from build123d import *

# Parameters (mm, degrees)
CUT_EXTRUDE1_START    = 5.5
CUT_EXTRUDE1_DEPTH    = 10
SKETCH8_R             = 6
CUT_EXTRUDE4_DEPTH    = 6
CUT_EXTRUDE5_START    = 6
CUT_EXTRUDE5_DEPTH    = 2.5
FILLET1_R             = 0.3
CHAMFER1_SIZE         = 0.5
M3_TAPPED_HOLE1_D     = 2.5
M3_TAPPED_HOLE1_DEPTH = 6.748924226
M3_TAPPED_HOLE1_TIP   = 0.751075774


with BuildPart() as part:
    # Sketch3 → Revolve1 (revolve)
    with BuildSketch(Plane.XY):
        Polygon((-10, 9), (10, 9), (10, 6), (32, 6), (60, 6), (60, 0), (-30, 0), (-30, 6), (-10, 6), align=None)
    revolve(axis=Axis((-30, 0, 0), (1, 0, 0)))

    # Sketch5 → Cut-Extrude1 (cut)
    with BuildSketch(Plane(origin=(0, 0, 0), x_dir=(1, 0, 0), z_dir=(0, 1, 0)).offset(CUT_EXTRUDE1_START)):
        with BuildLine():
            Line((5, -3), (-5, -3))
            ThreePointArc((-5, -3), (-8, 0), (-5, 3))
            Line((-5, 3), (5, 3))
            ThreePointArc((5, 3), (8, 0), (5, -3))
        make_face()
    extrude(amount=CUT_EXTRUDE1_DEPTH, mode=Mode.SUBTRACT)

    # Sketch8 → Cut-Extrude4 (cut)
    with BuildSketch(Plane(origin=(60, 0, 0), x_dir=(0, 0, -1), z_dir=(1, 0, 0))):
        Circle(SKETCH8_R)
    extrude(amount=-CUT_EXTRUDE4_DEPTH, mode=Mode.SUBTRACT)

    # Sketch9 → Cut-Extrude5 (cut)
    with BuildSketch(Plane(origin=(0, 0, 0), x_dir=(1, 0, 0), z_dir=(0, 1, 0)).offset(CUT_EXTRUDE5_START)):
        with BuildLine():
            Line((42, 2), (48, 2))
            ThreePointArc((48, 2), (50, 0), (48, -2))
            Line((48, -2), (42, -2))
            ThreePointArc((42, -2), (40, 0), (42, 2))
        make_face()
    extrude(amount=-CUT_EXTRUDE5_DEPTH, mode=Mode.SUBTRACT)

    # Fillet1
    fillet1_edges = [part.edges().sort_by_distance(p)[0] for p in [
        (-10, -6, 0),
        (10, -6, 0),
    ]]
    fillet(fillet1_edges, radius=FILLET1_R)

    # Chamfer1
    chamfer1_edges = [part.edges().sort_by_distance(p)[0] for p in [
        (-30, -6, 0),
        (54, -6, 0),
    ]]
    chamfer(chamfer1_edges, length=CHAMFER1_SIZE)

    # M3 Tapped Hole1
    with Locations(Plane(origin=(54, 0, 0), x_dir=(0, 0, -1), z_dir=(1, 0, 0))):
        with Locations((0, 0)):
            Hole(M3_TAPPED_HOLE1_D / 2, depth=M3_TAPPED_HOLE1_DEPTH)
            with Locations((0, 0, -(M3_TAPPED_HOLE1_DEPTH + M3_TAPPED_HOLE1_TIP / 2))):  # 118° drill point
                Cone(0, M3_TAPPED_HOLE1_D / 2, M3_TAPPED_HOLE1_TIP, mode=Mode.SUBTRACT)


solid = part.part
The model under review builds one solid part; all positions refer to its coordinate system, in mm. A direction names the side the tool comes from. Round coordinates to 2 decimals unless told otherwise and drop trailing zeros. Loops run counter-clockwise (first coordinate to the right, second up) from the corner with the lowest first, then second, coordinate; pieces in that order, holes last. Notation, with made-up numbers: M 67.5,-15 L 105.5,-15 A29 cw 105.5,12 Z; hole C 53.5,45 d5. An arc over 180 degrees is marked long. Answer as a JSON object with one key per item and string values.
Item 1: Clearance check with flat-ended pins moving along their axes: P1, Ø2, axis at y = -6.5, z = 2, coming from the +X side; P2, Ø4.5, axis at x = 46.5, z = 1, coming from the +Y side; P3, Ø5, axis at x = 21.5, z = -3.5, coming from the -Y side. State where each tip first meets the part, or that it passes through.
Check sheet entries:
{"P1": "x = 53.7", "P2": "y = 5.68", "P3": "y = -5.92"}
Item 2: We need section B-B, the plane z = -7.5. State the section outline as (x, y) points, and give its area (3 significant figures).
Check sheet entries:
{"outline": "M -10,-4.97 L 10,-4.97 L 10,4.97 L -10,4.97 Z", "area": "199 mm2"}
Item 3: The part is to be moulded in two halves that separate along Z. For faces 4 (the face through (31.6, -4.76, -3.65)), 5 (the face through (54, -1, -1)), 6 (the face through (0, 5.5, 0)), say which applies: +Z half, -Z half, draft (parallel to the pull), parting line (faces both ways), or undercut.
Check sheet entries:
{"face 4": "parting line", "face 5": "draft", "face 6": "undercut"}
Item 4: We need section A-A, the plane x = -16. State the section outline as (y, z) points.
Check sheet entries:
{"outline": "C 0,0 d12"}
Item 5: Tool access review of faces 1 (the face through (-10, 6.1, 2.1)), 2 (the face through (45, 3.5, 0)), 3 (the face through (10, -6.1, 2.1)): name each direction out of +Z, -Z, +X, -X, +Y, -Y from which nothing blocks a thin tool from reaching the whole face with its end or side.
Check sheet entries:
{"face 1": "-X", "face 2": "+Y", "face 3": "+X"}
Item 6: For line 1 along Y through (x, z) = (49.25, 0); line 2 along Y through (x, z) = (50.75, 0), list the stretches that pass through material, from the lowest coordinate up.
Check sheet entries:
{"line 1": "-6 to -1.25, 1.25 to 3.5", "line 2": "-6 to -1.25, 1.25 to 6"}
